Autodesk Inventor part; units mm, degrees
ref_plane "YZ Plane" through (0, 0, 0) normal (1, 0, 0) x (0, 1, 0)
ref_plane "XZ Plane" through (0, 0, 0) normal (0, 1, 0) x (-1, 0, 0)
ref_plane "XY Plane" through (0, 0, 0) normal (0, 0, 1) x (1, 0, 0)
sketch "Esquisse1" plane through (0, 0, 0) normal (1, 0, 0) x (0, 1, 0)
  line L0 (0, 0) -> (5, 0)
  line L1 (5, 0) -> (5, -2)
  line L2 (5, -2) -> (3, -2)
  line L3 (3, -2) -> (3, -11)
  line L4 (3, -11) -> (0, -11)
  line L5 (0, -11) -> (0, 0)
  dimension "d1" = 2
  dimension "d2" = 9
  dimension "d3" = 3
  dimension "d4" = 5
revolve "Révolution1" add sketch "Esquisse1" angle 360 about axis through (0, 0, -11) along (0, 0, 1)
sketch "Esquisse2" plane through (0, 0, -11) normal (0, 0, -1) x (-1, 0, 0)
  point P0 (0, 0)
  point P1 (0, 0)
hole "Perçage1" at (0, 0, -11) direction (0, 0, 1) diameter 2.459 end through all
chamfer "Chanfrein1" distance 0.5 angle 45 1 edges at (0, -3, -11)
properties part number "axe_taraude_m4"
For this review, take the finished solid that the model builds, in its own axes (mm). A direction names the side the tool comes from. Give positions to 0.01 mm unless a question says otherwise; leave off trailing zeros. Loops run counter-clockwise (first coordinate to the right, second up) from the corner with the lowest first, then second, coordinate; pieces in that order, holes last. Notation, with made-up numbers: M 13,-8.5 L 29,-8.5 A16 ccw 29,-1.5 Z; hole C 53,-3.5 d2. An arc over 180 degrees is marked long. Answer as a JSON object with one key per item and string values. Group by question number.
Q1. Mouldability with a two-part tool opening along X and no side actions: class faces 3 (the cylindrical face through (0.748, -0.976, -5.423)), 4 (the flat face through (-1, 1, -11)), 5 (the cylindrical face through (-4.88, -1.08, -1.01)) as +X half, -X half, draft (parallel to the pull), parting line (faces both ways), or undercut.
Q2. Add section A-A on y = 0. Give the boundary of the cut face in (x, z).
Q3. Add section C-C on z = -6.75. Give the boundary of the cut face in (x, y).
Q4. Insertion check: P1, Ø5, axis at y = -1.5, z = -6.5, coming from the +X side. The pin has a flat end and moves straight along its axis. Give the tip position at first contact, or say it passes through.
Q5. Tool access review of faces 1 (the flat face through (1, 1, 0)), 2 (the flat face through (-0.1, 3.3, -2)): name each direction out of +Z, -Z, +X, -X, +Y, -Y from which nothing blocks a thin tool from reaching the whole face with its end or side.
Q6. For probe 1 along X at (y, z) = (0, -6.75); probe 2 along Z at (x, y) = (1, -3), list the stretches that pass through material, from the lowest coordinate up. Write a range as [from, to].
Q7. Add section D-D on y = 4. Give the boundary of the cut face in (x, z), and give its area (3 significant figures).
Checked values:
{
 "1": {"face 3": "undercut", "face 4": "draft", "face 5": "parting line"},
 "2": {"outline": "M -5,-2 L -3,-2 L -3,-10.5 L -2.5,-11 L -1.23,-11 L -1.23,0 L -5,0 Z; M 1.23,-11 L 2.5,-11 L 3,-10.5 L 3,-2 L 5,-2 L 5,0 L 1.23,0 Z"},
 "3": {"outline": "C 0,0 d6; hole C 0,0 d2.46"},
 "4": {"P1": "x = 3"},
 "5": {"face 1": "+Z, +X, -X, +Y, -Y", "face 2": "-Z"},
 "6": {"probe 1": "[-3, -1.23], [1.23, 3]", "probe 2": "[-2, 0]"},
 "7": {"outline": "M -3,-2 L 3,-2 L 3,0 L -3,0 Z", "area": "12.0 mm²"}
}
